from build123d import *

# Parameters (mm, degrees)
SKETCH015_W  = 105.6
SKETCH015_H  = 20.8
PAD005_DEPTH = 3
SKETCH016_R  = 3
PAD006_DEPTH = 3
SKETCH017_R  = 1.75
PAD007_DEPTH = 3


with BuildPart() as part:
    # Sketch015 → Pad005 (new body)
    with BuildSketch(Plane.XZ.offset(-104)):
        with Locations((96.000001, 16.4)):
            Rectangle(SKETCH015_W, SKETCH015_H)
    extrude(amount=PAD005_DEPTH)

    # Sketch016 (on Face1 of Pad005) → Pad006 (join)
    with BuildSketch(Plane(origin=(0, 0, 26.8), x_dir=(-1, 0, 0), z_dir=(0, 0, 1))):
        with BuildLine():
            ThreePointArc((-92.000001, -96.00002), (-95.999992, -92), (-100.000001, -96.000001))
            Line((-100.000001, -96.000001), (-100.000001, -101))
            Line((-100.000001, -101), (-92.000001, -101))
            Line((-92.000001, -96.00002), (-92.000001, -101))
        make_face()
        with Locations((-96.000001, -96)):
            Circle(SKETCH016_R, mode=Mode.SUBTRACT)
    extrude(amount=-PAD006_DEPTH)

    # Sketch017 (on Face11 of Pad006) → Pad007 (join)
    with BuildSketch(Plane(origin=(0, 0, 26.8), x_dir=(-1, 0, 0), z_dir=(0, 0, 1))):
        with BuildLine():
            Line((-92.000001, -96.00002), (-92.000001, -100.60001))
            Line((-92.000001, -100.60001), (-100.000001, -100.6))
            Line((-100.000001, -100.6), (-100.000001, -96.000001))
            ThreePointArc((-92.000001, -96.00002), (-95.999992, -92.000035), (-100.000001, -96.000001))
        make_face()
        with Locations((-96.000001, -96)):
            Circle(SKETCH017_R, mode=Mode.SUBTRACT)
    extrude(amount=PAD007_DEPTH)


solid = part.part
Geometry check sheet. Reference: the model listing, model coordinates, mm. A direction names the side the tool comes from. Coordinates: 2 decimals unless noted, no trailing zeros. Order: outer loops, then holes, each group sorted by start corner. A loop starts at its lowest first (then second) coordinate and runs counter-clockwise, first axis right, second up. Notation, with made-up numbers: (1, 62) - (18, 62) arc R18 cw to (18, 79) - close; hole circle Ø4 at (-37, -4). An arc over 180 degrees is marked (long way). Answer in a Markdown table with one row per item. Add a question column.
1) Gauge pin test, flat ends, axial feed: P1, Ø5, axis at x = 96, y = 96, coming from the -Z side; P2, Ø5.5, axis at y = 97.5, z = 27, coming from the +X side; P3, Ø5, axis at x = 64, z = 16, coming from the -Y side; P4, Ø3, axis at x = 96, y = 96, coming from the +Z side. Record the tip position at first contact, or that the pin passes through.
2) Release check for a two-part mould opening along Y. For faces 1 (the cylindrical face through (96, 92, 28)), 2 (the flat face through (98, 96, 26.8)), 3 (the cylindrical face through (97.39, 97.06, 28.28)), 4 (the flat face through (148.8, 103, 16)) record: +Y half, -Y half, draft (parallel to the pull), parting line (faces both ways), or undercut.
3) Material ranges on line 1 along Y through (x, z) = (96, 28.7); line 2 along Y through (x, z) = (65.5, 16.5); line 3 along Y through (x, z) = (96, 24.7), recorded low to high. Write a range as [from, to].
4) Set-up check for faces 5 (the flat face through (95, 102, 26.8)), 6 (the flat face through (100, 99, 27)), 7 (the flat face through (92, 98, 27)), 8 (the flat face through (96.1, 99.4, 23.8)): record each of +Z, -Z, +X, -X, +Y, -Y from which the full face is reachable in a straight line by a thin tool's end or side.
5) Cross-section at A-A, the plane z = 13.5. Record the cut outline in (x, y), then the cut area to 3 significant figures.
6) Cross-section at B-B, the plane x = 84.5. Record the cut outline in (y, z).
Check result:
| question | item | result |
|---|---|---|
| 1 | P1 | stops at z = 26.8 |
| 1 | P2 | stops at x = 100 |
| 1 | P3 | stops at y = 101 |
| 1 | P4 | passes through |
| 2 | face 1 | -Y half |
| 2 | face 2 | undercut |
| 2 | face 3 | undercut |
| 2 | face 4 | draft |
| 3 | line 1 | y = [92, 94.25], [97.75, 100.6] |
| 3 | line 2 | y = [101, 104] |
| 3 | line 3 | y = [92, 93], [99, 104] |
| 4 | face 5 | +Z, +X, -X, +Y |
| 4 | face 6 | +Z, -Z, +X, -Y |
| 4 | face 7 | +Z, -Z, -X, -Y |
| 4 | face 8 | -Z, +X, -X, -Y |
| 5 | outline | (43.2, 101) - (148.8, 101) - (148.8, 104) - (43.2, 104) - close |
| 5 | area | 317 mm² |
| 6 | outline | (101, 6) - (104, 6) - (104, 26.8) - (101, 26.8) - close |
